Geometry check sheet. Reference: the model listing, model coordinates, mm. A direction names the side the tool comes from. Round coordinates to 2 decimals unless told otherwise and drop trailing zeros. Order: outer loops, then holes, each group sorted by start corner. A loop starts at its lowest first (then second) coordinate and runs counter-clockwise, first axis right, second up.
```python
from build123d import *

# Parameters (mm, degrees)
F0_W     = 4.2091126258
F0_H     = 23.15
F1_DEPTH = 7.611
F2_W     = 2.1045563129
F2_H     = 7.611
F2_W_2   = 5.5041293296
F3_DEPTH = 2
F4_W     = 4.8296524825
F4_H     = 7.611
F4_W_2   = 2.1045563129
F5_DEPTH = 2
F6_W     = 2.1045563129
F6_H     = 7.611
F6_W_2   = 5.5243599842
F7_DEPTH = 2
F8_W     = 2.1045563129
F8_H     = 7.611
F8_W_2   = 4.695874514
F9_DEPTH = 2


with BuildPart() as f1:
    # F0 (on Front) → F1 (new body)
    with BuildSketch(Plane.XZ):
        Rectangle(F0_W, F0_H)
    extrude(amount=F1_DEPTH)

    # F2 (on face) → F3 (join)
    with BuildSketch(Plane.XY.offset(11.575)):
        with Locations((1.0522781564, -3.8055)):
            Rectangle(F2_W, F2_H)
        with Locations((4.8566209777, -3.8055)):
            Rectangle(F2_W_2, F2_H)
    extrude(amount=F3_DEPTH)

    # F4 (on face) → F5 (join)
    with BuildSketch(Plane.XY.offset(11.575)):
        with Locations((-4.5193825542, -3.8055)):
            Rectangle(F4_W, F4_H)
        with Locations((-1.0522781564, -3.8055)):
            Rectangle(F4_W_2, F4_H)
    extrude(amount=F5_DEPTH)

    # F6 (on face) → F7 (join)
    with BuildSketch(Plane(origin=(0, 0, -11.575), x_dir=(1, 0, 0), z_dir=(0, 0, -1))):
        with Locations((1.0522781564, 3.8055)):
            Rectangle(F6_W, F6_H)
        with Locations((4.866736305, 3.8055)):
            Rectangle(F6_W_2, F6_H)
    extrude(amount=F7_DEPTH)

    # F8 (on face) → F9 (join)
    with BuildSketch(Plane(origin=(0, 0, -11.575), x_dir=(1, 0, 0), z_dir=(0, 0, -1))):
        with Locations((-1.0522781564, 3.8055)):
            Rectangle(F8_W, F8_H)
        with Locations((-4.4524935699, 3.8055)):
            Rectangle(F8_W_2, F8_H)
    extrude(amount=F9_DEPTH)


solid = f1.part
```
(1) Set-up check for faces 1 (the flat face through (7.609, -4, 13)), 2 (the flat face through (-2.105, -4, 0)), 3 (the flat face through (5, -4, 11.575)): record each of +Z, -Z, +X, -X, +Y, -Y from which the full face is reachable in a straight line by a thin tool's end or side.
Returned:
face 1: +Z, +X, +Y, -Y
face 2: -X, +Y, -Y
face 3: +X, +Y, -Y
(2) Draft check along Z on faces 4 (the flat face through (-5, -4, 11.575)), 5 (the flat face through (-6.8, -4, -13)), 6 (the flat face through (0, -4, 13.575)). Enter one of: released by +Z, released by -Z, zero draft, split by the parting line, or undercut.
Returned:
face 4: undercut
face 5: zero draft
face 6: released by +Z
(3) Material ranges on line 1 (Z direction, x = 4, y = -6) (3 decimals); line 2 (X direction, y = -2, z = 11); line 3 (X direction, y = -6, z = -12.5), recorded low to high.
Returned:
line 1: z = -13.575 to -11.575, 11.575 to 13.575
line 2: x = -2.1 to 2.1
line 3: x = -6.8 to 7.63
(4) Sectioned sample at A-A, the plane x = -2.75. Record the cut outline in (y, z) (3 decimals), and give its area (3 significant figures).
Returned:
outline: (-7.611, -13.575) - (0, -13.575) - (0, -11.575) - (-7.611, -11.575) - close; (-7.611, 11.575) - (0, 11.575) - (0, 13.575) - (-7.611, 13.575) - close
area: 30.4 mm2
(5) Sectioned sample at B-B, the plane y = -5. Record the cut outline in (x, z) (3 decimals).
Returned:
outline: (-6.934, 11.575) - (-2.105, 11.575) - (-2.105, -11.575) - (-6.8, -11.575) - (-6.8, -13.575) - (7.629, -13.575) - (7.629, -11.575) - (2.105, -11.575) - (2.105, 11.575) - (7.609, 11.575) - (7.609, 13.575) - (-6.934, 13.575) - close
(6) Depth check by flat-ended pin: P1, Ø2, axis at y = -5, z = -12.5, coming from the -X side; P2, Ø2.5, axis at y = -4.5, z = -1.5, coming from the -X side; P3, Ø1, axis at y = -5.5, z = 12.5, coming from the +X side. Enter the tip coordinate at first touch or a pass-through.
Returned:
P1: stops at x = -6.8
P2: stops at x = -2.1
P3: stops at x = 7.61
(7) Sectioned sample at C-C, the plane z = 5.5. Record the cut outline in (x, y), and give its area (3 significant figures).
Returned:
outline: (-2.1, -7.61) - (2.1, -7.61) - (2.1, 0) - (-2.1, 0) - close
area: 32.0 mm2
